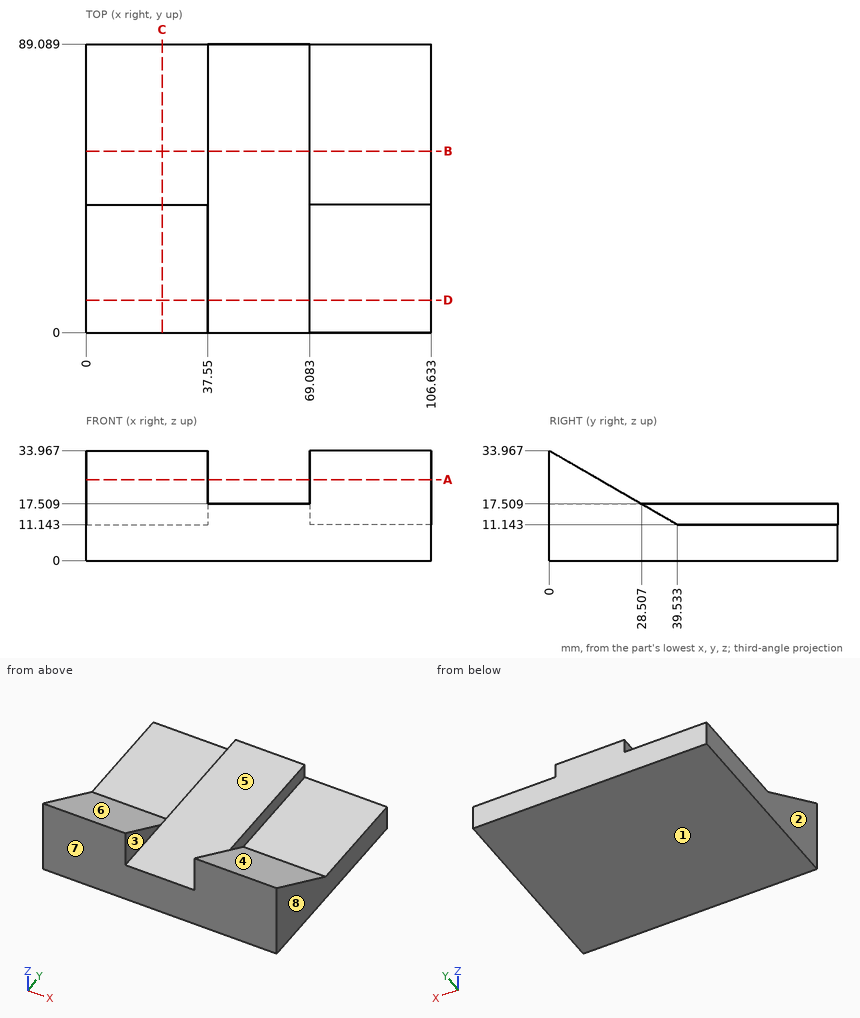
Drawing for the job (mm, zero at the part's lowest x, y, z). A direction names the side the tool comes from. Give positions to 0.01 mm unless a question says otherwise; leave off trailing zeros. Loops run counter-clockwise (first coordinate to the right, second up) from the corner with the lowest first, then second, coordinate; pieces in that order, holes last.
Item 1: Drop flat-ended pins along their axis: P1, Ø9.5, axis at x = 59, y = 41, coming from the +Z side; P2, Ø5, axis at y = 48, z = 14, coming from the +X side; P3, Ø19, axis at x = 93, y = 60.5, coming from the +Z side; P4, Ø5, axis at y = 19, z = 26.5, coming from the -X side. Give the stop position or say it passes through.
Check values:
P1: stops at z = 17.51
P2: stops at x = 69.08
P3: stops at z = 11.14
P4: passes through
Item 2: Which spindle directions (+Z, -Z, +X, -X, +Y, -Y) get a long thin tool onto all of the face, cutting with end or side? Do the marked faces 4, 5, 6, 7 and 8. Say none if no direction does.
Check values:
face 4: +Z, +X, +Y
face 5: +Z, +Y, -Y
face 6: +Z, -X, +Y
face 7: +Z, -Z, +X, -X, -Y
face 8: +Z, -Z, +X, +Y, -Y
Item 3: Slice it at B-B (y = 56). Write the cut outline in (x, z).
Check values:
outline: (0, 0) - (106.63, 0) - (106.63, 11.14) - (69.08, 11.14) - (69.08, 17.51) - (37.55, 17.51) - (37.55, 11.14) - (0, 11.14) - close
Item 4: Mould opens along X. For the marked faces 1, 2 and 3 say: +X half, -X half, draft (parallel to the pull), parting line (faces both ways), or undercut.
Check values:
face 1: draft
face 2: -X half
face 3: undercut
Item 5: Slice it at C-C (x = 23.5). Write the cut outline in (y, z), plus the area to 3 significant figures.
Check values:
outline: (0, 0) - (89.09, 0) - (89.09, 11.14) - (39.53, 11.14) - (0, 33.97) - close
area: 1,440 mm2
Item 6: Slice it at D-D (y = 10). Write the cut outline in (x, z), plus the area to 3 significant figures.
Check values:
outline: (0, 0) - (106.63, 0) - (106.63, 28.19) - (69.08, 28.19) - (69.08, 17.51) - (37.55, 17.51) - (37.55, 28.19) - (0, 28.19) - close
area: 2,670 mm2
Item 7: Drill centre lines: line 1 along Z through (x, y) = (56, 20); line 2 along X through (y, z) = (17, 23); line 3 along Z through (x, y) = (77, 42). Where is each one in solid material? Low to high.
Check values:
line 1: z = 0 to 17.51
line 2: x = 0 to 37.55, 69.08 to 106.63
line 3: z = 0 to 11.14
Item 8: Slice it at A-A (z = 25). Write the cut outline in (x, y).
Check values:
outline: (0, 0) - (37.55, 0) - (37.55, 15.53) - (0, 15.53) - close; (69.08, 0) - (106.63, 0) - (106.63, 15.53) - (69.08, 15.53) - close
